Source: CAD feature listing. Evaluate the final solid. Frame: model axes, mm. A direction names the side the tool comes from. Coordinates: 2 decimals unless noted, no trailing zeros. Order: outer loops, then holes, each group sorted by start corner. A loop starts at its lowest first (then second) coordinate and runs counter-clockwise, first axis right, second up.
```python
from build123d import *

# Parameters (mm, degrees)
BOSS_EXTRU_1_DEPTH           = 6.5
ENL_V_MAT_EXTRU_1_DEPTH      = 20
ENL_V_MAT_EXTRU_1_DEPTH_BACK = 33.283896915
ESQUISSE4_W                  = 20
ESQUISSE4_H                  = 7
ESQUISSE5_R                  = 5
ENL_V_MAT_EXTRU_2_DEPTH      = 35.190641995


with BuildPart() as part:
    # Esquisse3 → Boss.-Extru.1 (new, symmetric)
    with BuildSketch(Plane(origin=(0, 0, 0), x_dir=(1, 0, 0), z_dir=(0, 1, 0))):
        with BuildLine():
            Line((-10, -30), (-10, 0))
            ThreePointArc((-10, 0), (0, 10), (10, 0))
            Line((10, 0), (10, -30))
            Line((10, -30), (-10, -30))
        make_face()
    extrude(amount=BOSS_EXTRU_1_DEPTH, both=True)

    # Esquisse4 → Enlèv. mat.-Extru.1 (cut, two sides: drawn at the far end of the back side and taken through both)
    with BuildSketch(Plane.XY.offset(-ENL_V_MAT_EXTRU_1_DEPTH_BACK)):
        Rectangle(ESQUISSE4_W, ESQUISSE4_H)
    extrude(amount=ENL_V_MAT_EXTRU_1_DEPTH + ENL_V_MAT_EXTRU_1_DEPTH_BACK, mode=Mode.SUBTRACT)

    # Esquisse5 → Enlèv. mat.-Extru.2 (cut, through all)
    with BuildSketch(Plane(origin=(0, 6.5, 0), x_dir=(1, 0, 0), z_dir=(0, 1, 0))):
        with Locations(Location((0, 0, 0), (0, 0, 270))):
            Circle(ESQUISSE5_R)
    extrude(amount=-ENL_V_MAT_EXTRU_2_DEPTH, mode=Mode.SUBTRACT)


solid = part.part
```
1. Section query C-C on y = 5.25. Return loops of the section in (x, z), plus the area to 3 significant figures.
Findings:
outline: (-10, 0) arc R10 ccw to (10, 0) - (10, 30) - (-10, 30) - close; hole circle Ø10 at (0, 0)
area: 679 mm2
2. Draft query along Y for faces 1 (the face through (0, 0, 30)), 2 (the face through (0, -6.5, 14)), 3 (the face through (0, 3.5, 8)). Return one class per face: released by +Y, released by -Y, zero draft, split by the parting line, or undercut.
Findings:
face 1: zero draft
face 2: released by -Y
face 3: undercut
3. Section query B-B on x = 0. Return loops of the section in (y, z), plus the area to 3 significant figures.
Findings:
outline: (-6.5, -10) - (-3.5, -10) - (-3.5, -5) - (-6.5, -5) - close; (-6.5, 5) - (-3.5, 5) - (-3.5, 20) - (3.5, 20) - (3.5, 5) - (6.5, 5) - (6.5, 30) - (-6.5, 30) - close; (3.5, -10) - (6.5, -10) - (6.5, -5) - (3.5, -5) - close
area: 250 mm2
4. Ray query, line 1 (Y direction, x = -5, z = 2); line 2 (X direction, y = -4.85, z = 0); line 3 (Z direction, x = 3, y = -1.75). Return the intervals inside material, ascending.
Findings:
line 1: y = -6.5 to -3.5, 3.5 to 6.5
line 2: x = -10 to -5, 5 to 10
line 3: z = 20 to 30
5. Section query A-A on z = 8. Return loops of the section in (x, y).
Findings:
outline: (-10, -6.5) - (10, -6.5) - (10, -3.5) - (-10, -3.5) - close; (-10, 3.5) - (10, 3.5) - (10, 6.5) - (-10, 6.5) - close
6. Section query D-D on z = 1. Return loops of the section in (x, y).
Findings:
outline: (-10, -6.5) - (-4.9, -6.5) - (-4.9, -3.5) - (-10, -3.5) - close; (-10, 3.5) - (-4.9, 3.5) - (-4.9, 6.5) - (-10, 6.5) - close; (4.9, -6.5) - (10, -6.5) - (10, -3.5) - (4.9, -3.5) - close; (4.9, 3.5) - (10, 3.5) - (10, 6.5) - (4.9, 6.5) - close
7. Pin query (flat end, axial travel): P1, Ø2, axis at x = 7, y = -1.5, coming from the -Z side. Return the tip coordinate at first contact, or that it passes through.
Findings:
P1: stops at z = 20
8. Access query for faces 4 (the face through (-10, 0, 22)), 5 (the face through (0, 0, 20)). Directions: +Z, -Z, +X, -X, +Y, -Y. A direction counts if a zero-diameter tool reaches every point of the face in a straight line with its end or side. Return the directions, or none.
Findings:
face 4: +Z, -Z, -X, +Y, -Y
face 5: -Z, +X, -X
